from build123d import *

# Parameters (mm, degrees)
F0_W     = 50.8
F0_H     = 50.8
F1_DEPTH = 101.6
F3_DEPTH = 99.06
F4_DEPTH = 99.06


with BuildPart() as f1:
    # F0 (on Top) → F1 (new body)
    with BuildSketch(Plane.XY):
        with Locations((25.4, 25.4)):
            Rectangle(F0_W, F0_H)
    extrude(amount=F1_DEPTH)

    # F2 (on face) → F3 (cut)
    with BuildSketch(Plane.XY.offset(101.6)):
        Polygon((2.54, 7.489045), (2.54, 2.545525), (18.157401, 2.54), (47.233673, 2.529714), (22.108479, 26.818483), (2.54, 45.735521), align=None)
    extrude(amount=-F3_DEPTH, mode=Mode.SUBTRACT)

    # F2 (on face) → F4 (cut)
    with BuildSketch(Plane.XY.offset(101.6)):
        Polygon((3.224171, 48.606943), (23.873876, 28.644674), (48.26, 5.070372), (48.26, 33.179211), (48.26, 48.151647), (37.52937, 48.26013), align=None)
    extrude(amount=-F4_DEPTH, mode=Mode.SUBTRACT)


solid = f1.part
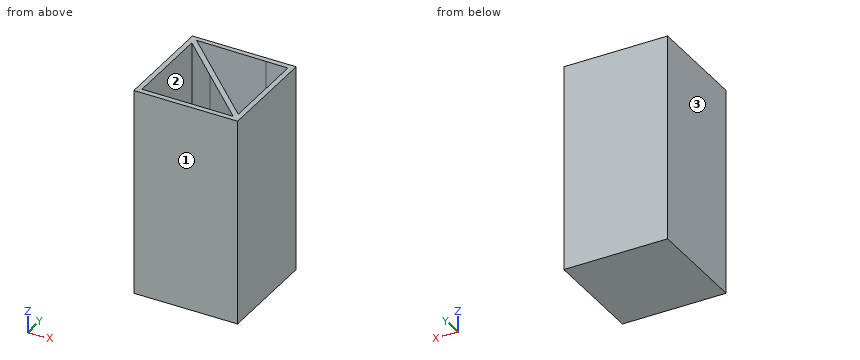
Design review of the part built by this model. Coordinates are the model's own, in mm. Face numbers are marked on the shaded views. Give positions to 0.01 mm unless a question says otherwise; leave off trailing zeros. Loops run counter-clockwise (first coordinate to the right, second up) from the corner with the lowest first, then second, coordinate; pieces in that order, holes last. Notation, with made-up numbers: (-33.75, -28) -> (-21.75, -28) arc R10 ccw to (-21.75, -9) -> close; hole circle Ø1 at (69, 53). An arc over 180 degrees is marked (long way). One line per question, with ' | ' between items. Start each with the question number.
(1) We need section C-C (x = 43). State the section outline as (y, z) points, and give its area (3 significant figures).
(2) We need section B-B (y = 8). State the section outline as (x, z) points (3 decimals), and give its area (3 significant figures).
(3) Draft analysis for pull direction Y (two halves, no side actions). For the marked faces 1, 2 and 3, state which applies: +Y half, -Y half, draft (parallel to the pull), parting line (faces both ways), or undercut.
(4) For line 1 (X direction, y = 44.5, z = 75); line 2 (Y direction, x = 9, z = 95); line 3 (X direction, y = 37, z = 75), list the stretches that pass through material, from the lowest coordinate up.
(5) We need section A-A (z = 83.5). State the section outline as (x, y) points.
The answers:
1) outline: (0, 0) -> (50.8, 0) -> (50.8, 101.6) -> (48.2, 101.6) -> (48.2, 2.54) -> (10.16, 2.54) -> (10.16, 101.6) -> (6.62, 101.6) -> (6.62, 2.54) -> (2.53, 2.54) -> (2.53, 101.6) -> (0, 101.6) -> close | area: 987 mm^2
2) outline: (0, 0) -> (50.8, 0) -> (50.8, 101.6) -> (48.26, 101.6) -> (48.26, 2.54) -> (45.229, 2.54) -> (45.229, 101.6) -> (41.575, 101.6) -> (41.575, 2.54) -> (2.54, 2.54) -> (2.54, 101.6) -> (0, 101.6) -> close | area: 994 mm^2
3) face 1: -Y half | face 2: undercut | face 3: draft
4) line 1: x = 0 to 2.54, 3.82 to 7.47, 48.26 to 50.8 | line 2: y = 0 to 2.54, 39.49 to 43.02, 48.55 to 50.8 | line 3: x = 0 to 2.54, 11.58 to 15.23, 48.26 to 50.8
5) outline: (0, 0) -> (50.8, 0) -> (50.8, 50.8) -> (0, 50.8) -> close; hole (2.54, 2.55) -> (47.23, 2.53) -> (2.54, 45.74) -> close; hole (3.22, 48.61) -> (48.26, 5.07) -> (48.26, 48.15) -> close
